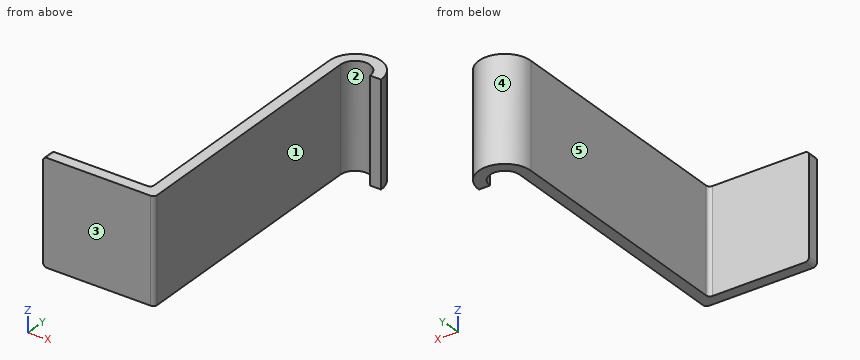
```python
from build123d import *

# Parameters (mm, degrees)
BOSS_EXTRUDE1_DEPTH = 28
FILLET1_R           = 1


with BuildPart() as part:
    # Sketch1 → Boss-Extrude1 (new body)
    with BuildSketch(Plane.XY):
        with BuildLine():
            Line((0, 0), (0, -70))
            Line((0, -70), (-30, -70))
            Line((-30, -70), (-30, -67))
            Line((-30, -67), (-3, -67))
            Line((-3, -67), (-3, 0))
            ThreePointArc((-3, 0), (4, 7), (11, 0))
            Line((11, 0), (8, 0))
            ThreePointArc((8, 0), (4, 4), (0, 0))
        make_face()
    extrude(amount=BOSS_EXTRUDE1_DEPTH)

    # Fillet1
    fillet1_edges = [part.edges().sort_by_distance(p)[0] for p in [
        (0, -70, 14),
        (-3, -67, 14),
        (-30, -68.5, 28),
        (-30, -68.5, 0),
    ]]
    fillet(fillet1_edges, radius=FILLET1_R)


solid = part.part
```
CAD build for the part. Positions are in the model's coordinates, mm. Face numbers are marked on the shaded views. A direction names the side the tool comes from. Coordinates: 2 decimals unless noted, no trailing zeros. Order: outer loops, then holes, each group sorted by start corner. A loop starts at its lowest first (then second) coordinate and runs counter-clockwise, first axis right, second up. Notation, with made-up numbers: M 49.5,72.5 L 103.5,72.5 A17 ccw 103.5,88.5 Z; hole C 35,3 d9. An arc over 180 degrees is marked long. Answer as CSV lines item,"result".
1) Cut at B-B (x = 4). List the corners of the cut face in (y, z), then the cut area to 3 significant figures.
Verdict:
outline,"M 4,0 L 7,0 L 7,28 L 4,28 Z"
area,"84.0 mm2"
2) Mould opens along X. For the marked faces 1, 2 and 3 say: released by +X, released by -X, zero draft, split by the parting line, or undercut.
Verdict:
face 1,"released by +X"
face 2,"undercut"
face 3,"zero draft"
3) Flat gauge pins, fed straight in: P1, Ø3, axis at y = -59.5, z = 14, coming from the -X side; P2, Ø3, axis at y = -61.5, z = 17, coming from the +X side; P3, Ø12, axis at x = -14, y = -11.5, coming from the +Z side; P4, Ø10, axis at x = -10, z = 10, coming from the +Y side. Where does each tip first touch, or does it go through?
Verdict:
P1,"x = -3"
P2,"x = 0"
P3,"through"
P4,"y = -67"
4) Cut at A-A (z = 17). List the corners of the cut face in (x, y), then the cut area to 3 significant figures.
Verdict:
outline,"M -30,-70 L -1,-70 A1 ccw 0,-69 L 0,0 A4 cw 8,0 L 11,0 A7 ccw -3,0 L -3,-66 A1 cw -4,-67 L -30,-67 Z"
area,"343 mm2"
5) Drill centre lines: L1, parallel to X at y = -56, z = 3; L2, parallel to Y at x = -12.5, z = 10.5; L3, parallel to X at y = 3, z = 3.75. Where is each one in solid material? Low to high. Write a range as from..to.
Verdict:
L1,"-3..0"
L2,"-70..-67"
L3,"-2.32..1.35, 6.65..10.32"
6) Cut at C-C (y = -28). List the corners of the cut face in (x, z), then the cut area to 3 significant figures.
Verdict:
outline,"M -3,0 L 0,0 L 0,28 L -3,28 Z"
area,"84.0 mm2"
7) 3-axis set-ups, long thin cutter, end or side, ignore diameter. For the marked faces 4 and 5: which of +Z, -Z, +X, -X, +Y, -Y reach the whole face in a straight line?
Verdict:
face 4,"+Z, -Z, +Y"
face 5,"+Z, -Z, -X, +Y"
